Geometry: final body of the model. Coordinates: model frame, mm. A direction names the side the tool comes from. Coordinates: 2 decimals unless noted, no trailing zeros. Write each loop counter-clockwise with the first axis right and the second up, starting at its lowest first coordinate (ties: lowest second). Pieces come first, ordered by that corner, then holes. Notation, with made-up numbers: (-23, 87.5) - (23, 87.5) arc R4 cw to (23, 94.5) - close; hole circle Ø9 at (12.25, 1.5). An arc over 180 degrees is marked (long way). Put each result on its own line as item: value.
```python
from build123d import *

# Parameters (mm, degrees)
F0_R     = 9.4326970336
F0_R_2   = 5
F1_DEPTH = 11
F0_R_3   = 17.5
F0_R_4   = 14.1231381544
F2_START = 0.5
F2_DEPTH = 10


with BuildPart() as f1:
    # F0 (on Top) → F1 (new body)
    with BuildSketch(Plane.XY):
        Circle(F0_R)
        Circle(F0_R_2, mode=Mode.SUBTRACT)
    extrude(amount=F1_DEPTH)



with BuildPart() as f1b:
    # F0 (on Top) → F1, piece 2 (new body)
    with BuildSketch(Plane.XY):
        Circle(F0_R_3)
        Circle(F0_R_4, mode=Mode.SUBTRACT)
    extrude(amount=F1_DEPTH)


with BuildPart() as f1_1:
    add(f1.part)

    add(f1b.part)  # F2 merges F1b
    # F0 (on Top) → F2 (join)
    with BuildSketch(Plane.XY.offset(F2_START)):
        Circle(F0_R_4)
        Circle(F0_R, mode=Mode.SUBTRACT)
    extrude(amount=F2_DEPTH)


solid = f1_1.part
```
1. Set-up query: faces 1 (the flat face through (-12, 8, 11)), 2 (the flat face through (2.9, -9.2, 10.5)), 3 (the flat face through (2.9, -9.2, 0.5)). Return all of +Z, -Z, +X, -X, +Y, -Y with unobstructed straight access to the full face (end or side cutting, diameter ignored); none if empty.
Answer below:
face 1: +Z, +X, -X, +Y, -Y
face 2: +Z
face 3: -Z
2. Section query A-A (x = 0). Return loops of the section in (y, z), then the cut area to 3 significant figures.
Answer below:
outline: (-17.5, 0) - (-14.12, 0) - (-14.12, 0.5) - (-9.43, 0.5) - (-9.43, 0) - (-5, 0) - (-5, 11) - (-9.43, 11) - (-9.43, 10.5) - (-14.12, 10.5) - (-14.12, 11) - (-17.5, 11) - close; (5, 0) - (9.43, 0) - (9.43, 0.5) - (14.12, 0.5) - (14.12, 0) - (17.5, 0) - (17.5, 11) - (14.12, 11) - (14.12, 10.5) - (9.43, 10.5) - (9.43, 11) - (5, 11) - close
area: 266 mm²
3. Pin query (flat end, axial travel): pin 1 Ø2 at (x, z) = (-5, 1.5) entering from +Y; pin 2 Ø3 at (y, z) = (-5.5, 5) entering from +X; pin 3 Ø1 at (x, z) = (-9.5, 5) entering from +Y. Return the tip coordinate at first contact, or that it passes through.
Answer below:
pin 1: stops at y = 17.04
pin 2: stops at x = 17.04
pin 3: stops at y = 15.01
4. Section query C-C (z = 4.25). Return loops of the section in (x, y), then the cut area to 3 significant figures.
Answer below:
outline: circle Ø35 at (0, 0); hole circle Ø10 at (0, 0)
area: 884 mm²
5. Ray query, probe 1 along Y at (x, z) = (0, 10.8); probe 2 along Y at (x, z) = (0, 2.5); probe 3 along Z at (x, y) = (1, -10). Return the intervals inside material, ascending. Write a range as from..to.
Answer below:
probe 1: y = -17.5..-14.12, -9.43..-5, 5..9.43, 14.12..17.5
probe 2: y = -17.5..-5, 5..17.5
probe 3: z = 0.5..10.5
6. Section query D-D (x = 11). Return loops of the section in (y, z).
Answer below:
outline: (-13.61, 0) - (-8.86, 0) - (-8.86, 0.5) - (8.86, 0.5) - (8.86, 0) - (13.61, 0) - (13.61, 11) - (8.86, 11) - (8.86, 10.5) - (-8.86, 10.5) - (-8.86, 11) - (-13.61, 11) - close
7. Mould query, pull axis Y, two halves, no side actions, for faces 4 (the cylindrical face through (-7.485, -5.74, 0.246)), 5 (the flat face through (-12, 8, 0)), 6 (the cylindrical face through (-13.887, -10.648, 5.423)). Classes: +Y half, -Y half, draft (parallel to the pull), parting line (faces both ways), or undercut.
Answer below:
face 4: undercut
face 5: draft
face 6: parting line
